Here's how the part is built. I have some questions about the finished solid (model axes, mm). Coordinates: 2 decimals unless noted, no trailing zeros. Write each loop counter-clockwise with the first axis right and the second up, starting at its lowest first coordinate (ties: lowest second). Pieces come first, ordered by that corner, then holes.
Item 1: If we section it at B-B (z = 1.2): Please give me the cut outline in (x, y), then the cut area to 3 significant figures.
Item 2: If I drill on line 1 (X direction, y = 11, z = 1); line 2 (X direction, y = 11.5, z = 3.2); line 3 (Y direction, x = 12, z = 4.65), over which ranges is the centre line in solid material (lowest first)?
Item 3: I'm going to push flat-ended pins straight in: pin 1 Ø1.5 at (x, y) = (-15.5, -8.5) entering from -Z; pin 2 Ø1.8 at (x, y) = (12.12, -19.45) entering from +Z. Where does each tip first touch, or does it pass through?
Item 4: If we section it at A-A (x = 13): Please give me the cut outline in (y, z).
from build123d import *

# Parameters (mm, degrees)
F0_W     = 36
F0_H     = 36
F1_DEPTH = 5
F2_D     = 3
F3_R     = 4


with BuildPart() as f1:
    # F0 (on Top) → F1 (new body)
    with BuildSketch(Plane.XY):
        with Locations((-3.1273178756, -4.2013906179)):
            Rectangle(F0_W, F0_H)
    extrude(amount=F1_DEPTH)

    # F2 (through all)
    with Locations(Plane(origin=(0, 0, 0), x_dir=(1, 0, 0), z_dir=(0, 0, -1))):
        with Locations((12.1226821244, -11.0486093821), (-18.3773178756, -11.0486093821), (-18.3773178756, 19.4513906179), (12.1226821244, 19.4513906179)):
            Hole(F2_D / 2)

    # F3
    f3_edges = [f1.edges().sort_by_distance(p)[0] for p in [
        (14.872682, -22.201391, 2.5),
        (14.872682, 13.798609, 2.5),
        (-21.127318, -22.201391, 2.5),
        (-21.127318, 13.798609, 2.5),
    ]]
    fillet(f3_edges, radius=F3_R)


solid = f1.part
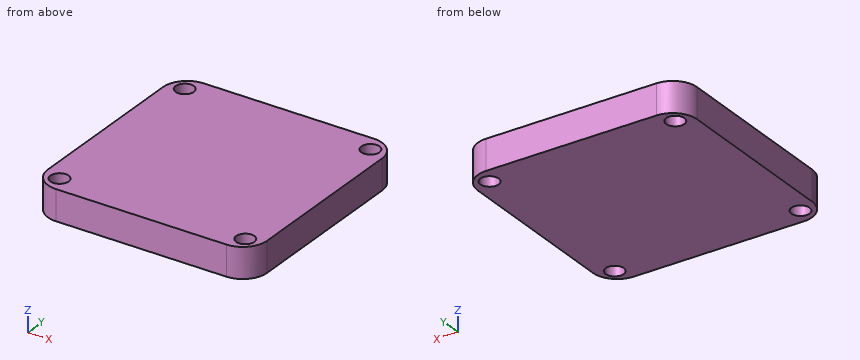
Answer list:
1. outline: (-21.13, -18.2) arc R4 ccw to (-17.13, -22.2) - (10.87, -22.2) arc R4 ccw to (14.87, -18.2) - (14.87, 9.8) arc R4 ccw to (10.87, 13.8) - (-17.13, 13.8) arc R4 ccw to (-21.13, 9.8) - close; hole circle Ø3 at (-18.38, -19.45); hole circle Ø3 at (-18.38, 11.05); hole circle Ø3 at (12.12, -19.45); hole circle Ø3 at (12.12, 11.05)
1. area: 1,250 mm2
2. line 1: x = -20.94 to -19.88, -16.88 to 10.62, 13.62 to 14.69
2. line 2: x = -20.75 to -19.81, -16.95 to 10.69, 13.55 to 14.49
2. line 3: y = -22.04 to -20.95, -17.96 to 9.55, 12.54 to 13.64
3. pin 1: stops at z = 0
3. pin 2: passes through
4. outline: (-21.59, 0) - (-20.67, 0) - (-20.67, 5) - (-21.59, 5) - close; (-18.23, 0) - (9.83, 0) - (9.83, 5) - (-18.23, 5) - close; (12.27, 0) - (13.19, 0) - (13.19, 5) - (12.27, 5) - close
